Check sheet for the modelled part. Datum: model origin and axes. Units: mm. A direction names the side the tool comes from. Coordinates: 2 decimals unless noted, no trailing zeros. Order: outer loops, then holes, each group sorted by start corner. A loop starts at its lowest first (then second) coordinate and runs counter-clockwise, first axis right, second up.
1. Thickness scan on line 1 (X direction, y = 4, z = 24.5); line 2 (X direction, y = 2, z = -22.5); line 3 (X direction, y = 2, z = -25.5). Record the ranges inside material, lowest first.
2. Cross-section at A-A (x = 0). Enter the section's corners in (y, z), then the cut area to 3 significant figures.
3. Cross-section at B-B (z = 0). Enter the section's corners in (x, y).
4. Cross-section at C-C (y = 9.5). Count the separate pieces of the cut face and the enclosed holes in it, then the cut area to 3 significant figures.
5. Draft check along Y on faces 6 (the cylindrical face through (0.08, 20.13, 40.43)), 7 (the cylindrical face through (-35.757, 9.042, -7.12)), 8 (the conical face through (0.092, 35.615, 34.667)), 9 (the cylindrical face through (38.48, 32.13, 12.41)). Enter one of: released by +Y, released by -Y, zero draft, split by the parting line, or undercut.
6. Gauge pin test, flat ends, axial feed: pin 1 Ø8 at (x, z) = (22.5, -17) entering from +Y; pin 2 Ø5.5 at (x, z) = (0, -32) entering from +Y; pin 3 Ø8 at (x, y) = (9, 13) entering from +Z; pin 4 Ø6 at (y, z) = (14.5, 15.5) entering from +X. Record the tip position at first contact, or that the pin passes through.
7. Set-up check for faces 1 (the flat face through (6, 25, 38)), 2 (the flat face through (38.1, 24.82, 6.07)), 3 (the flat face through (-6, 25, 38)), 4 (the conical face through (-32.942, 35.615, 10.8)), 5 (the flat face through (-17.732, 6.084, -14.198)): record each of +Z, -Z, +X, -X, +Y, -Y from which the full face is reachable in a straight line by a thin tool's end or side.
```python
from build123d import *

# Parameters (mm, degrees)
CUT_EXTRUDE_2_DEPTH      = 69.74590907246773
SKETCH_6_R               = 3.000000000000353
SKETCH_6_R_2             = 9.5
SKETCH_6_R_3             = 3.0000000000000013
SKETCH_6_R_4             = 3.0000000000001754
SKETCH_6_R_5             = 3.0000000000002696
SKETCH_6_R_6             = 3.0000000000000875
CUT_EXTRUDE_3_DEPTH      = 69.74590907417861
SKETCH_7_R               = 5.999999999999999
SKETCH_7_R_2             = 3.0000000000000013
SKETCH_7_R_3             = 6.0000000000003535
SKETCH_7_R_4             = 3.000000000000353
SKETCH_7_R_5             = 6.00000000000009
SKETCH_7_R_6             = 3.0000000000000875
SKETCH_7_R_7             = 6.000000000000174
SKETCH_7_R_8             = 3.0000000000001754
SKETCH_7_R_9             = 6.00000000000027
SKETCH_7_R_10            = 3.000000000000269
CUT_EXTRUDE_4_DEPTH      = 6
CUT_EXTRUDE_5_REACH      = 81.273
SKETCH_8_R               = 3.0000000000000018
PATTERN_CIRCULAR_1_COUNT = 5


with BuildPart() as part:
    # Sketch 2 → Revolve 1 (revolve)
    with BuildSketch(Plane(origin=(0, 0, 0), x_dir=(0, 0, -1), z_dir=(1, 0, 0))):
        with BuildLine():
            Line((0, 0), (-45, -6.94e-15))
            Line((-45, -6.94e-15), (-45, 33))
            ThreePointArc((-45, 33), (-42.454374247383356, 37.35615048566752), (-37.40958117848744, 37.27664942789954))
            Line((-37.40958117848744, 37.27664942789954), (-31.99999999999998, 34))
            Line((-31.99999999999998, 34), (-31.999999999999993, 12))
            Line((-31.999999999999993, 12), (3.86e-15, 12))
            Line((3.86e-15, 12), (0, 0))
        make_face()
    revolve(axis=Axis((0, 43.5345852345433, 0), (0, -1, 0)))

    # Sketch 3 → Cut-Extrude 2 (cut, through all)
    with BuildSketch(Plane(origin=(0, 12, 0), x_dir=(1, 0, 0), z_dir=(0, 1, 0))):
        with BuildLine():
            Line((6.000000000000002, -12.649110640673518), (6.000000000000003, -44.59820624195551))
            ThreePointArc((6.000000000000003, -44.59820624195551), (26.450336353161088, -36.40576474687278), (40.561312695237085, -19.48794274517449))
            Line((40.561312695237085, -19.48794274517449), (10.175917133901121, -9.615129249468135))
            ThreePointArc((10.175917133901121, -9.615129249468135), (8.228993532094561, -11.326237921249312), (6.000000000000002, -12.649110640673518))
        make_face()
        with BuildLine():
            Line((-5.999999999999998, -12.649110640673518), (-5.999999999999992, -44.59820624195551))
            ThreePointArc((-5.999999999999992, -44.59820624195551), (-26.45033635316134, -36.405764746872606), (-40.56131269523736, -19.487942745173925))
            Line((-40.56131269523736, -19.487942745173925), (-10.175917133901258, -9.61512924946799))
            ThreePointArc((-10.175917133901258, -9.61512924946799), (-8.228993532094645, -11.326237921249254), (-5.999999999999998, -12.649110640673518))
        make_face()
        with BuildLine():
            Line((-13.884121066400596, 1.7975489460738636), (-44.2695166277367, -8.075264549632074))
            ThreePointArc((-44.2695166277367, -8.075264549632074), (-42.797543233281836, 13.905764746872823), (-31.068269873969072, 32.553995254626194))
            Line((-31.068269873969072, 32.553995254626194), (-12.289062655453339, 6.706633958279081))
            ThreePointArc((-12.289062655453339, 6.706633958279081), (-13.314791228132133, 4.3262379212493185), (-13.884121066400596, 1.7975489460738636))
        make_face()
        with BuildLine():
            Line((-2.5808587229539293, 13.760056985788705), (-21.36006594146967, 39.60741828213582))
            ThreePointArc((-21.36006594146967, 39.60741828213582), (3.225e-13, 44.999999999999986), (21.360065941470232, 39.60741828213551))
            Line((21.360065941470232, 39.60741828213551), (2.5808587229541256, 13.760056985788673))
            ThreePointArc((2.5808587229541256, 13.760056985788673), (1.0033e-13, 14.000000000000002), (-2.5808587229539293, 13.760056985788705))
        make_face()
        with BuildLine():
            Line((12.289062655453431, 6.70663395827891), (31.068269873969538, 32.55399525462576))
            ThreePointArc((31.068269873969538, 32.55399525462576), (42.79754323328205, 13.905764746872206), (44.26951662773658, -8.075264549632692))
            Line((44.26951662773658, -8.075264549632692), (13.88412106640062, 1.797548946073666))
            ThreePointArc((13.88412106640062, 1.797548946073666), (13.314791228132195, 4.32623792124913), (12.289062655453431, 6.70663395827891))
        make_face()
    extrude(amount=CUT_EXTRUDE_2_DEPTH, mode=Mode.SUBTRACT)

    # Sketch 6 → Cut-Extrude 3 (cut, through all)
    with BuildSketch(Plane(origin=(0, 12, 0), x_dir=(1, 0, 0), z_dir=(0, 1, 0))):
        with BuildLine():
            ThreePointArc((12.289062655453431, 6.7066339582789105), (8.228993532094725, 11.326237921249191), (2.580858722954132, 13.760056985788669))
            Line((2.580858722954132, 13.760056985788669), (13.62143875056792, 28.956111727311136))
            ThreePointArc((13.62143875056792, 28.956111727311136), (18.809128073359357, 25.888543819998144), (23.329642683067217, 21.90268869980138))
            Line((23.329642683067217, 21.90268869980138), (12.289062655453431, 6.7066339582789105))
        make_face()
        with BuildLine():
            ThreePointArc((10.175917133901127, -9.615129249468133), (13.314791228132105, -4.326237921249419), (13.88412106640062, 1.7975489460736591))
            Line((13.88412106640062, 1.7975489460736591), (31.7481548065927, -4.006827470284166))
            ThreePointArc((31.7481548065927, -4.006827470284166), (30.433808521444792, -9.888543819998658), (28.039950874093208, -15.419505665825957))
            Line((28.039950874093208, -15.419505665825957), (10.175917133901127, -9.615129249468133))
        make_face()
        with BuildLine():
            ThreePointArc((-5.999999999999995, -12.649110640673522), (8.6e-16, -14.000000000000002), (5.999999999999995, -12.649110640673522))
            Line((5.999999999999995, -12.649110640673522), (5.999999999999995, -31.43246729100341))
            ThreePointArc((5.999999999999995, -31.43246729100341), (1.96e-15, -31.999999999999986), (-5.999999999999995, -31.43246729100341))
            Line((-5.999999999999995, -31.43246729100341), (-5.999999999999995, -12.649110640673522))
        make_face()
        with BuildLine():
            ThreePointArc((-13.884121066400597, 1.7975489460738576), (-13.314791228132165, -4.326237921249228), (-10.175917133901264, -9.615129249467987))
            Line((-10.175917133901264, -9.615129249467987), (-28.03995087409343, -15.419505665825561))
            ThreePointArc((-28.03995087409343, -15.419505665825561), (-30.43380852144493, -9.888543819998239), (-31.748154806592765, -4.006827470283715))
            Line((-31.748154806592765, -4.006827470283715), (-13.884121066400597, 1.7975489460738576))
        make_face()
        with BuildLine():
            ThreePointArc((-2.5808587229539373, 13.760056985788708), (-8.228993532094563, 11.326237921249309), (-12.289062655453337, 6.706633958279092))
            Line((-12.289062655453337, 6.706633958279092), (-23.32964268306691, 21.902688699801722))
            ThreePointArc((-23.32964268306691, 21.902688699801722), (-18.80912807335899, 25.888543819998407), (-13.621438750567506, 28.956111727311335))
            Line((-13.621438750567506, 28.956111727311335), (-2.5808587229539373, 13.760056985788708))
        make_face()
        with Locations(Location((-30.433808521444917, 9.888543819998311, 0), (0, 0, 270))):
            Circle(SKETCH_6_R)
        with Locations(Location((0, 0, 0), (0, 0, 270))):
            Circle(SKETCH_6_R_2)
        with Locations(Location((0, 32, 0), (0, 0, 270))):
            Circle(SKETCH_6_R_3)
        with Locations(Location((18.809128073359144, -25.888543819998315, 0), (0, 0, 270))):
            Circle(SKETCH_6_R_4)
        with Locations(Location((-18.80912807335914, -25.888543819998322, 0), (0, 0, 270))):
            Circle(SKETCH_6_R_5)
        with Locations(Location((30.433808521444917, 9.888543819998324, 0), (0, 0, 270))):
            Circle(SKETCH_6_R_6)
    extrude(amount=-CUT_EXTRUDE_3_DEPTH, mode=Mode.SUBTRACT)

    # Sketch 7 → Cut-Extrude 4 (cut)
    # profile 1 of 5: a face of its own
    with BuildSketch(Plane(origin=(0, 12, 0), x_dir=(1, 0, 0), z_dir=(0, 1, 0))):
        with Locations(Location((0, 32, 0), (0, 0, 270))):
            Circle(SKETCH_7_R)
        with Locations(Location((0, 32, 0), (0, 0, 270))):
            Circle(SKETCH_7_R_2, mode=Mode.SUBTRACT)
    # profile 2 of 5: a face of its own
    with BuildSketch(Plane(origin=(0, 12, 0), x_dir=(1, 0, 0), z_dir=(0, 1, 0))):
        with Locations(Location((-30.433808521444917, 9.888543819998311, 0), (0, 0, 270))):
            Circle(SKETCH_7_R_3)
        with Locations(Location((-30.433808521444917, 9.888543819998311, 0), (0, 0, 270))):
            Circle(SKETCH_7_R_4, mode=Mode.SUBTRACT)
    # profile 3 of 5: a face of its own
    with BuildSketch(Plane(origin=(0, 12, 0), x_dir=(1, 0, 0), z_dir=(0, 1, 0))):
        with Locations(Location((30.433808521444917, 9.888543819998324, 0), (0, 0, 270))):
            Circle(SKETCH_7_R_5)
        with Locations(Location((30.433808521444917, 9.888543819998324, 0), (0, 0, 270))):
            Circle(SKETCH_7_R_6, mode=Mode.SUBTRACT)
    # profile 4 of 5: a face of its own
    with BuildSketch(Plane(origin=(0, 12, 0), x_dir=(1, 0, 0), z_dir=(0, 1, 0))):
        with Locations(Location((18.809128073359144, -25.888543819998315, 0), (0, 0, 270))):
            Circle(SKETCH_7_R_7)
        with Locations(Location((18.809128073359144, -25.888543819998315, 0), (0, 0, 270))):
            Circle(SKETCH_7_R_8, mode=Mode.SUBTRACT)
    # profile 5 of 5: a face of its own
    with BuildSketch(Plane(origin=(0, 12, 0), x_dir=(1, 0, 0), z_dir=(0, 1, 0))):
        with Locations(Location((-18.80912807335914, -25.888543819998322, 0), (0, 0, 270))):
            Circle(SKETCH_7_R_9)
        with Locations(Location((-18.80912807335914, -25.888543819998322, 0), (0, 0, 270))):
            Circle(SKETCH_7_R_10, mode=Mode.SUBTRACT)
    extrude(amount=-CUT_EXTRUDE_4_DEPTH, mode=Mode.SUBTRACT)

    # Sketch 8 → Cut-Extrude 5 (cut, up to next)
    with BuildSketch(Plane(origin=(-4.854101966249707, 0, 3.5267115137548144), x_dir=(0.5877852522924687, 0, 0.8090169943749507), z_dir=(-0.8090169943749507, 0, 0.5877852522924687)), mode=Mode.PRIVATE) as cut_extrude_5_sk1:
        with Locations((-37.4324672910034, 32)):
            Circle(SKETCH_8_R)
    cut_extrude_5_tool1 = extrude(cut_extrude_5_sk1.sketch, amount=-CUT_EXTRUDE_5_REACH, mode=Mode.PRIVATE) & part.part
    # Sketch 8 → Cut-Extrude 5 (cut, up to next)
    with BuildSketch(Plane(origin=(-4.854101966249707, 0, 3.5267115137548144), x_dir=(0.5877852522924687, 0, 0.8090169943749507), z_dir=(-0.8090169943749507, 0, 0.5877852522924687)), mode=Mode.PRIVATE) as cut_extrude_5_sk2:
        with Locations((-37.4324672910034, 19.999999999999993)):
            Circle(SKETCH_8_R)
    cut_extrude_5_tool2 = extrude(cut_extrude_5_sk2.sketch, amount=-CUT_EXTRUDE_5_REACH, mode=Mode.PRIVATE) & part.part
    cut_extrude_5_1 = cut_extrude_5_tool1.solids().sort_by_distance((-26.856354, 32, -26.756791))[0]
    add(cut_extrude_5_1, mode=Mode.SUBTRACT)
    cut_extrude_5_2 = cut_extrude_5_tool2.solids().sort_by_distance((-26.856354, 20, -26.756791))[0]
    add(cut_extrude_5_2, mode=Mode.SUBTRACT)
    cut_extrude_5 = cut_extrude_5_1 + cut_extrude_5_2  # Cut-Extrude 5 as one shape, for the pattern or mirror that repeats it

    # Pattern Circular 1: Cut-Extrude 5 ×5 about axis
    pattern_circular_1_axis = Axis((0, 12, 0), (0, 1, 0))
    for i in range(1, PATTERN_CIRCULAR_1_COUNT):
        add(cut_extrude_5.rotate(pattern_circular_1_axis, i * 360 / PATTERN_CIRCULAR_1_COUNT), mode=Mode.SUBTRACT)


solid = part.part
```
Data:
1. line 1: x = -37.75 to -21.47, -16.15 to -6, 6 to 16.15, 21.47 to 37.75
1. line 2: x = -38.97 to -22.75, -8.93 to 8.93, 22.75 to 38.97
1. line 3: x = -37.08 to -19.33, -11.11 to 11.11, 19.33 to 37.08
2. outline: (0, -45) - (12, -45) - (12, -38) - (6, -38) - (6, -35) - (0, -35) - close; (0, -29) - (6, -29) - (6, -26) - (12, -26) - (12, -9.5) - (0, -9.5) - close; (0, 9.5) - (12, 9.5) - (12, 14) - (0, 14) - close; (0, 32) - (34, 32) - (37.28, 37.41) arc R5 ccw to (33, 45) - (0, 45) - close; hole circle Ø6 at (20, 37.43); hole circle Ø6 at (32, 37.43)
2. area: 791 mm2
3. outline: (-45, 0) - (-19.42, 0) - (-19.42, 12) - (-45, 12) - close; (-14, 0) - (-9.5, 0) - (-9.5, 12) - (-14, 12) - close; (9.5, 0) - (14, 0) - (14, 12) - (9.5, 12) - close; (19.42, 0) - (45, 0) - (45, 12) - (19.42, 12) - close
4. separate pieces: 1
4. enclosed holes: 11
4. area: 4,420 mm2
5. face 6: undercut
5. face 7: zero draft
5. face 8: released by +Y
5. face 9: undercut
6. pin 1: stops at y = 12
6. pin 2: passes through
6. pin 3: stops at z = 44.72
6. pin 4: stops at x = 43.23
7. face 1: +Z, -Z, +X, +Y
7. face 2: -Z, +X, +Y
7. face 3: +Z, -Z, -X, +Y
7. face 4: +Y
7. face 5: +Y, -Y
